Read the model definition and answer for the solid it produces. Units are mm, in the model's axes. A direction names the side the tool comes from. Round coordinates to 2 decimals unless told otherwise and drop trailing zeros. Order: outer loops, then holes, each group sorted by start corner. A loop starts at its lowest first (then second) coordinate and runs counter-clockwise, first axis right, second up. Notation, with made-up numbers: (-30.75, 49) -> (16.25, 49) arc R15 cw to (16.25, 68) -> close; hole circle Ø11 at (-22, 15). An arc over 180 degrees is marked (long way). Use a Markdown table: item, result. Add a question column.
1. Consider L1, parallel to X at y = 0, z = 1.1; L2, parallel to X at y = 9.5, z = 3.5; L3, parallel to Y at x = -2.5, z = 0.2. Determine where each line is inside the solid, lowest interval first. Write a range as [from, to].
2. Given pin 1 (1 mm diameter, centred on x = -2.5, z = 2.5, fed in from +Y), flat-ended and moving along its own axis, determine where the tip first touches the part or whether it passes through.
3. Section A-A, the plane y = 0 is taken. Give the vertices of the cut face in (x, z), then the cut area to 3 significant figures.
4. Section C-C, the plane x = 0 is taken. Give the vertices of the cut face in (y, z), then the cut area to 3 significant figures.
5. For faces 5 (the face through (7.928, 3.275, 1.878)), 6 (the face through (9.964, 14.015, 1.878)), 7 (the face through (-12.7, -1, 2)), determine the directions among +Z, -Z, +X, -X, +Y, -Y from which every point of the face is accessible in a straight line to the end or side of a thin tool.
6. The mould has two halves that part along Y. Classify faces 1 (the face through (0, -9, 0)), 2 (the face through (-12.21, 13.91, 1.88)), 3 (the face through (-7.928, 3.275, 1.878)), 4 (the face through (0.227, -8.506, 1.878)): +Y half, -Y half, draft (parallel to the pull), parting line (faces both ways), or undercut.
7. Section B-B, the plane z = 2.6 is taken. Give the vertices of the cut face in (x, y) (1 decimal).
8. Section D-D, the plane y = 11.25 is taken. Give the vertices of the cut face in (x, z).
```python
from build123d import *

# Parameters (mm, degrees)
F1_DEPTH    = 3.81
F2_T1_DEPTH = 11.945118529
F2_T3_DEPTH = 13.335
F2_T5_DEPTH = 6.3475490509


# Not quite as in the source:
# - a fillet or chamfer that OpenCascade refuses, or shapes differently, is made with other operations: its cross-section is extruded or revolved along the edge and cut away or added


with BuildPart() as f1:
    # F0 (on Top) → F1 (new body)
    with BuildSketch(Plane.XY):
        with BuildLine():
            ThreePointArc((7.8636785966, 3.2504830303), (0, -8.509), (-7.8636785966, 3.2504830303))
            Line((-7.8636785966, 3.2504830303), (-9.652, 14.5415))
            Line((-9.652, 14.5415), (-12.7, 14.5415))
            Line((-12.7, 14.5415), (-12.7, -14.5415))
            Line((-12.7, -14.5415), (12.7, -14.5415))
            Line((12.7, -14.5415), (12.7, 14.5415))
            Line((12.7, 14.5415), (9.652, 14.5415))
            Line((9.652, 14.5415), (7.8636785966, 3.2504830303))
        make_face()
    extrude(amount=F1_DEPTH)

    # F2: fillet of radius 1.905 on 6 edges, made by hand

    # F2_s2 → F2_t1 (cut)
    with BuildSketch(Plane.XY.offset(-4.0675592645)):
        with BuildLine():
            ThreePointArc((-9.397477417, 12.9345076559), (-10.0418251737, 14.0850733645), (-11.2790237058, 14.5415))
            Line((-11.2790237058, 14.5415), (-9.652, 14.5415))
            Line((-9.652, 14.5415), (-9.397477417, 12.9345076559))
        make_face()
        with BuildLine():
            ThreePointArc((11.2790237058, 14.5415), (10.0418251737, 14.0850733645), (9.397477417, 12.9345076559))
            Line((9.397477417, 12.9345076559), (9.652, 14.5415))
            Line((9.652, 14.5415), (11.2790237058, 14.5415))
        make_face()
    extrude(amount=F2_T1_DEPTH, mode=Mode.SUBTRACT)

    # F2_s4 → F2_t3 (cut)
    with BuildSketch(Plane.XY.offset(-4.7625)):
        with BuildLine():
            ThreePointArc((-10.795, 14.5415), (-12.1420384182, 13.9835384182), (-12.7, 12.6365))
            Line((-12.7, 12.6365), (-12.7, 14.5415))
            Line((-12.7, 14.5415), (-10.795, 14.5415))
        make_face()
        with BuildLine():
            ThreePointArc((12.7, 12.6365), (12.1420384182, 13.9835384182), (10.795, 14.5415))
            Line((10.795, 14.5415), (12.7, 14.5415))
            Line((12.7, 14.5415), (12.7, 12.6365))
        make_face()
    extrude(amount=F2_T3_DEPTH, mode=Mode.SUBTRACT)

    # F2_s6 → F2_t5 (cut)
    with BuildSketch(Plane.XY.offset(-1.2687745255)):
        with BuildLine():
            ThreePointArc((-8.0274308907, 2.821955757), (-7.9274098449, 3.2816022158), (-7.9430706222, 3.7517445525))
            Line((-7.9430706222, 3.7517445525), (-7.8636785966, 3.2504830303))
            ThreePointArc((-7.8636785966, 3.2504830303), (-7.9484431866, 3.0373231487), (-8.0274308907, 2.821955757))
        make_face()
        with BuildLine():
            ThreePointArc((8.0274308907, 2.821955757), (7.9274098449, 3.2816022158), (7.9430706222, 3.7517445525))
            Line((7.9430706222, 3.7517445525), (7.8636785966, 3.2504830303))
            ThreePointArc((7.8636785966, 3.2504830303), (7.9484431866, 3.0373231487), (8.0274308907, 2.821955757))
        make_face()
    extrude(amount=F2_T5_DEPTH, mode=Mode.SUBTRACT)


solid = f1.part
```
Verdict:
| question | item | result |
|---|---|---|
| 1 | L1 | x = [-12.7, -8.51], [8.51, 12.7] |
| 1 | L2 | x = [-12.7, -8.85], [8.85, 12.7] |
| 1 | L3 | y = [-14.54, -8.13] |
| 2 | pin 1 | stops at y = -7.96 |
| 3 | outline | (-12.7, 0) -> (-8.51, 0) -> (-8.51, 3.81) -> (-12.7, 3.81) -> close; (8.51, 0) -> (12.7, 0) -> (12.7, 3.81) -> (8.51, 3.81) -> close |
| 3 | area | 31.9 mm2 |
| 4 | outline | (-14.54, 0) -> (-8.51, 0) -> (-8.51, 3.81) -> (-14.54, 3.81) -> close |
| 4 | area | 23.0 mm2 |
| 5 | face 5 | +Z, -Z |
| 5 | face 6 | +Z, -Z, +Y |
| 5 | face 7 | +Z, -Z, -X, +Y, -Y |
| 6 | face 1 | draft |
| 6 | face 2 | +Y half |
| 6 | face 3 | undercut |
| 6 | face 4 | undercut |
| 7 | outline | (-12.7, -14.5) -> (12.7, -14.5) -> (12.7, 12.6) arc R1.9 ccw to (11, 14.5) arc R1.9 ccw to (9.4, 12.9) -> (7.9, 3.8) arc R1.9 ccw to (8, 2.8) arc R8.5 cw (long way) to (-8, 2.8) arc R1.9 ccw to (-7.9, 3.8) -> (-9.4, 12.9) arc R1.9 ccw to (-11, 14.5) arc R1.9 ccw to (-12.7, 12.6) -> close |
| 8 | outline | (-12.7, 0) -> (-9.13, 0) -> (-9.13, 3.81) -> (-12.7, 3.81) -> close; (9.13, 0) -> (12.7, 0) -> (12.7, 3.81) -> (9.13, 3.81) -> close |
